Can you work these out from the drawing? Everything is in mm from the part's minimum corner. A direction names the side the tool comes from. Coordinates: 2 decimals unless noted, no trailing zeros. Loops run counter-clockwise (first coordinate to the right, second up) from the corner with the lowest first, then second, coordinate; pieces in that order, holes last.
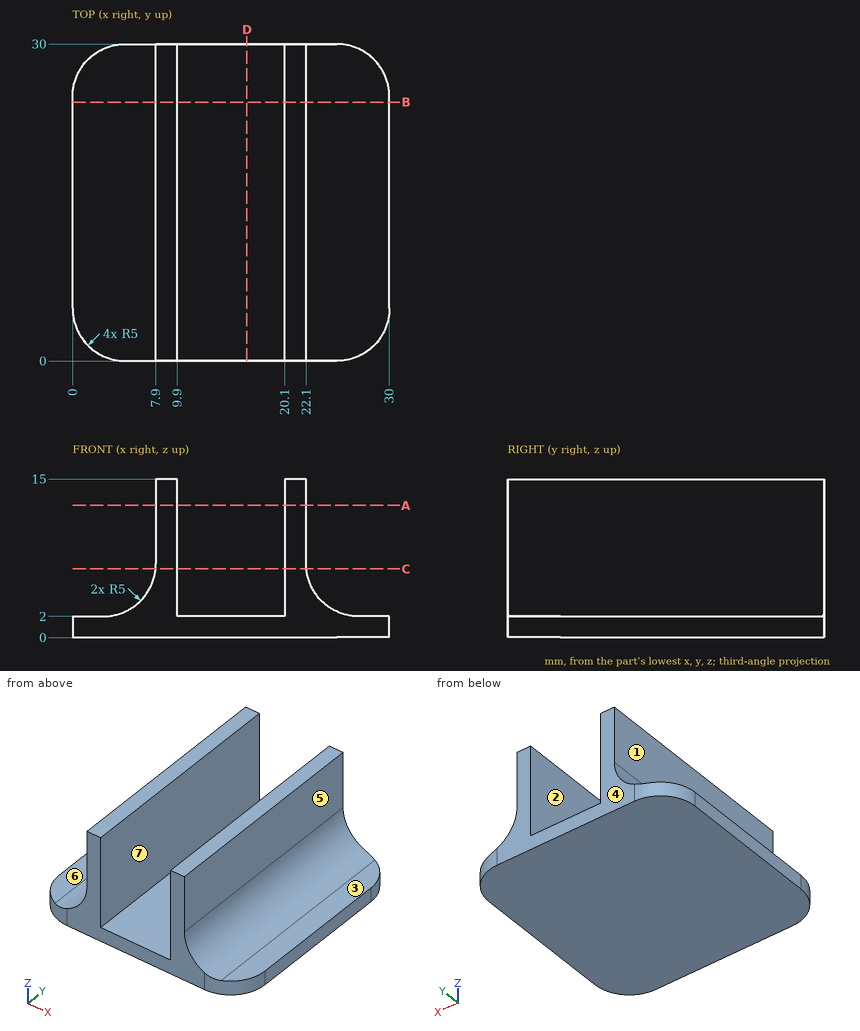
Item 1: Suppose I cut it at D-D, the plane x = 16.5. Please give me the cut outline in (y, z), plus the area to 3 significant figures.
Results are:
outline: (0, 0) - (30, 0) - (30, 2) - (0, 2) - close
area: 60.0 mm2
Item 2: Suppose I cut it at A-A, the plane z = 12.5. Please give me the cut outline in (x, y), plus the area to 3 significant figures.
Results are:
outline: (7.9, 0) - (9.9, 0) - (9.9, 30) - (7.9, 30) - close; (20.1, 0) - (22.1, 0) - (22.1, 30) - (20.1, 30) - close
area: 120 mm2
Item 3: I'm going to push flat-ended pins straight in: P1, Ø5, axis at y = 3, z = 10, coming from the +X side; P2, Ø8, axis at y = 10.5, z = 5, coming from the +X side; P3, Ø9, axis at y = 19.5, z = 9, coming from the -X side; P4, Ø2, axis at x = 13, y = 8, coming from the +Z side. Where does each tip first touch, or does it pass through?
Results are:
P1: stops at x = 22.1
P2: stops at x = 30
P3: stops at x = 7.23
P4: stops at z = 2
Item 4: Suppose I cut it at C-C, the plane z = 6.5. Please give me the cut outline in (x, y).
Results are:
outline: (7.87, 0) - (9.9, 0) - (9.9, 30) - (7.87, 30) - close; (20.1, 0) - (22.13, 0) - (22.13, 30) - (20.1, 30) - close
Item 5: Suppose I cut it at B-B, the plane y = 24.5. Please give me the cut outline in (x, z).
Results are:
outline: (0, 0) - (30, 0) - (30, 2) - (27.1, 2) arc R5 cw to (22.1, 7) - (22.1, 15) - (20.1, 15) - (20.1, 2) - (9.9, 2) - (9.9, 15) - (7.9, 15) - (7.9, 7) arc R5 cw to (2.9, 2) - (0, 2) - close
Item 6: On a 3-axis mill with a long thin cutter (end or side, diameter ignored), from which of +Z, -Z, +X, -X, +Y, -Y can I reach the whole of each face in a straight line? I mean the marked faces 4, 5, 6 and 7. Say none if no direction works.
Results are:
face 4: +Z, -Z, +X, -X, +Y
face 5: +Z, +X, +Y, -Y
face 6: +Z, -X, +Y, -Y
face 7: +Z, +Y, -Y
Item 7: We'd pull the mould along X, two halves only. Please class the marked faces 1, 2 and 3: +X half, -X half, draft (parallel to the pull), parting line (faces both ways), or undercut.
Results are:
face 1: -X half
face 2: undercut
face 3: draft
Item 8: I need wall thicknesses on line 1 along X through (y, z) = (8.5, 9); line 2 along Z through (x, y) = (16, 9.5); line 3 along X through (y, z) = (22.5, 5.5). Which ranges of each line are inside material? Lowest first, please.
Results are:
line 1: x = 7.9 to 9.9, 20.1 to 22.1
line 2: z = 0 to 2
line 3: x = 7.67 to 9.9, 20.1 to 22.33
